CAD build for the part. Positions are in the model's coordinates, mm. A direction names the side the tool comes from. Round coordinates to 2 decimals unless told otherwise and drop trailing zeros. Order: outer loops, then holes, each group sorted by start corner. A loop starts at its lowest first (then second) coordinate and runs counter-clockwise, first axis right, second up. Notation, with made-up numbers: (8.5, 30) -> (64.5, 30) arc R22 cw to (64.5, 63) -> close; hole circle Ø3 at (-17.5, 77). An arc over 180 degrees is marked (long way). Return JSON: item names as keys, results as strings. Group by question number.
Q1. Cut at C-C (x = 42.5). Write the cut outline in (y, z).
Q2. Which spindle directions (+Z, -Z, +X, -X, +Y, -Y) get a long thin tool onto all of the face, cutting with end or side? Do faces 4 (the flat face through (-12, 4, -2)), 5 (the cylindrical face through (141, 2, 0)), 6 (the cylindrical face through (44.85, 2.46, 0.05)). Say none if no direction does.
Q3. Flat gauge pins, fed straight in: pin 1 (4.5 mm diameter, centred on x = 13.5, z = -12, fed in from -Y); pin 2 (2.5 mm diameter, centred on x = -79.5, y = 3.5, fed in from +Z); pin 3 (2.5 mm diameter, centred on x = 106, y = 1.5, fed in from -Z). Where does each tip first touch, or does it go through?
Q4. Cut at B-B (x = 87). Write the cut outline in (y, z), then the cut area to 3 significant figures.
Q5. Mould opens along X. For faces 1 (the cylindrical face through (137.15, 2.46, -0.05)), 2 (the flat face through (75.512, 2.465, -10.913)), 3 (the flat face through (0, 2, -15.987)) say: +X half, -X half, draft (parallel to the pull), parting line (faces both ways), or undercut.
Q6. Cut at A-A (x = -64). Write the cut outline in (y, z), then the cut area to 3 significant figures.
Q7. Probe line 1 along X through (y, z) = (4.35, 0); line 2 along Z through (x, y) = (13.5, 4.3); line 3 along X through (y, z) = (3.5, 3.25). List the from-to ranges inside material, lowest first.
from build123d import *

# Parameters (mm, degrees)
SKETCH1_R           = 2.25
SKETCH1_R_2         = 1.65
BOSS_EXTRUDE1_DEPTH = 5
SKETCH3_R           = 3.75
SKETCH3_R_2         = 3
CUT_EXTRUDE1_DEPTH  = 4


with BuildPart() as part:
    # Sketch1 → Boss-Extrude1 (new body)
    with BuildSketch(Plane(origin=(0, 0, 0), x_dir=(1, 0, 0), z_dir=(0, 1, 0))):
        with BuildLine():
            Line((0, 15.986538484), (0, -10))
            Line((0, -10), (13.827888575, -10))
            Line((13.827888575, -10), (135.197796243, -5.996738834))
            ThreePointArc((135.197796243, -5.996738834), (140.998192557, -0.147261838), (135.491832862, 5.979807726))
            Line((135.491832862, 5.979807726), (13.827888575, 15.986538484))
            Line((13.827888575, 15.986538484), (0, 15.986538484))
        make_face()
        with Locations(Location((13.5, 0, 0), (0, 0, 270))):
            Circle(SKETCH1_R, mode=Mode.SUBTRACT)
        with BuildLine():
            ThreePointArc((47, -2.15), (44.85, 0), (47, 2.15))
            Line((47, 2.15), (135, 2.15))
            ThreePointArc((135, 2.15), (137.15, 0), (135, -2.15))
            Line((135, -2.15), (47, -2.15))
        make_face(mode=Mode.SUBTRACT)
        with Locations(Location((13.5, 12, 0), (0, 0, 270))):
            Circle(SKETCH1_R_2, mode=Mode.SUBTRACT)
    extrude(amount=BOSS_EXTRUDE1_DEPTH)

    # Mirror1: part across plane


with BuildPart() as part_1:
    add(part.part)
    add(part.part.mirror(Plane(origin=(0, 0, 0), x_dir=(0, 0, 1), z_dir=(1, 0, 0))))

    # Sketch3 → Cut-Extrude1 (cut)
    with BuildSketch(Plane(origin=(0, 0, 0), x_dir=(1, 0, 0), z_dir=(0, 1, 0))):
        with Locations(Location((13.5, 0, 0), (0, 0, 270))):
            Circle(SKETCH3_R)
        with Locations(Location((13.5, 12, 0), (0, 0, 270))):
            Circle(SKETCH3_R_2)
        Polygon((-9.169872981, 0), (-11.334936491, 3.75), (-15.665063509, 3.75), (-17.830127019, 0), (-15.665063509, -3.75), (-11.334936491, -3.75), align=None)
        Polygon((-10.035898385, 12), (-11.767949192, 15), (-15.232050808, 15), (-16.964101615, 12), (-15.232050808, 9), (-11.767949192, 9), align=None)
    extrude(amount=CUT_EXTRUDE1_DEPTH, mode=Mode.SUBTRACT)


solid = part_1.part
Solution:
{
 "1": {"outline": "(0, -13.63) -> (5, -13.63) -> (5, 9.05) -> (0, 9.05) -> close"},
 "2": {"face 4": "-Y", "face 5": "+X, +Y, -Y", "face 6": "+Y, -Y"},
 "3": {"pin 1": "stops at y = 4", "pin 2": "stops at z = 7.88", "pin 3": "stops at z = -8.51"},
 "4": {"outline": "(0, -9.97) -> (5, -9.97) -> (5, -2.15) -> (0, -2.15) -> close; (0, 2.15) -> (5, 2.15) -> (5, 7.59) -> (0, 7.59) -> close", "area": "66.3 mm²"},
 "5": {"face 1": "undercut", "face 2": "+X half", "face 3": "draft"},
 "6": {"outline": "(0, -11.86) -> (5, -11.86) -> (5, -2.15) -> (0, -2.15) -> close; (0, 2.15) -> (5, 2.15) -> (5, 8.35) -> (0, 8.35) -> close", "area": "79.5 mm²"},
 "7": {"line 1": "x = -141 to -137.15, -44.85 to -15.75, -11.25 to 11.25, 15.75 to 44.85, 137.15 to 141", "line 2": "z = -15.99 to -13.65, -10.35 to -2.25, 2.25 to 10", "line 3": "x = -140.04 to -15.95, -11.05 to 11.63, 15.37 to 140.04"}
}
